```python
from build123d import *

# Parameters (mm, degrees)
SKETCH2_W                    = 37
SKETCH2_H                    = 30
BASE_FLANGE1_DEPTH           = 0.635
EDGE_FLANGE1_STRIP_W         = 4.0132
EDGE_FLANGE1_STRIP_H         = 0.635
EDGE_FLANGE1_STRIP_CUT_DEPTH = 37
EDGE_FLANGE1_DEPTH           = 37
EDGE_FLANGE2_START           = -6.6891
EDGE_FLANGE2_DEPTH           = 5.3175
EDGE_FLANGE2_2_DEPTH         = 0.3175
EDGE_FLANGE2_START_2         = -6.3716
EDGE_FLANGE2_3_DEPTH         = 5
EDGE_FLANGE3_START           = -6.6891
EDGE_FLANGE3_DEPTH           = 5.3175
EDGE_FLANGE3_2_DEPTH         = 0.3175
EDGE_FLANGE3_START_2         = -6.3716
EDGE_FLANGE3_3_DEPTH         = 5
SKETCH14_R                   = 1.7
CUT_EXTRUDE1_DEPTH           = 10
FILLET1_R                    = 3
SKETCH15_R                   = 1.7
CUT_EXTRUDE2_DEPTH           = 10


# Read off the part's stored shape, not the designer's step: Edge-Flange2, Edge-Flange3
# Sheet-metal steps are written as plain solids
with BuildPart() as part:
    # Sketch2 → Base-Flange1 (new body)
    with BuildSketch(Plane(origin=(0, 0, 0), x_dir=(0, 0, -1), z_dir=(1, 0, 0))):
        with Locations((18.5, -15)):
            Rectangle(SKETCH2_W, SKETCH2_H)
    extrude(amount=-BASE_FLANGE1_DEPTH)

    # Edge-Flange1 strip (across the edge) → Edge-Flange1 strip cut (cut)
    with BuildSketch(Plane(origin=(-0.635, 0, 0), x_dir=(0, -1, 0), z_dir=(0, 0, -1))):
        with Locations((-1.27, -0.3175)):
            Rectangle(EDGE_FLANGE1_STRIP_W, EDGE_FLANGE1_STRIP_H)
    extrude(amount=EDGE_FLANGE1_STRIP_CUT_DEPTH, mode=Mode.SUBTRACT)

    # Edge-Flange1 section (across the edge) → Edge-Flange1 (add)
    with BuildSketch(Plane(origin=(-0.635, 0, 0), x_dir=(0, -1, 0), z_dir=(0, 0, -1))):
        with BuildLine():
            Line((-0.635, 0.7366), (-0.635, 22))
            Line((-0.635, 22), (0, 22))
            Line((0, 22), (0, 0.7366))
            ThreePointArc((0, 0.7366), (0.215745145, 0.215745145), (0.7366, 0))
            Line((0.7366, 0), (0.7366, -0.635))
            ThreePointArc((0.7366, -0.635), (-0.233267661, -0.233267661), (-0.635, 0.7366))
        make_face()
    extrude(amount=EDGE_FLANGE1_DEPTH)

    # Edge-Flange2 outline → Edge-Flange2 (cut)
    with BuildSketch(Plane.YZ.offset(EDGE_FLANGE2_START)):
        with BuildLine():
            Line((0, 0), (0, -0.214574936))
            ThreePointArc((0, -0.214574936), (0.465815718, -0.711688642), (0.635, -1.3716))
            Line((0.635, -1.3716), (0.635, 0))
            Line((0.635, 0), (0, 0))
        make_face()
    extrude(amount=EDGE_FLANGE2_DEPTH, mode=Mode.SUBTRACT)

    # Edge-Flange2 2 outline → Edge-Flange2 2 (cut)
    with BuildSketch(Plane.YZ.offset(EDGE_FLANGE2_START)):
        with BuildLine():
            ThreePointArc((0.635, -1.3716), (0.465815718, -0.711688642), (0, -0.214574936))
            Line((0, -0.214574936), (0, -1.6891))
            Line((0, -1.6891), (0.635, -1.6891))
            Line((0.635, -1.6891), (0.635, -1.3716))
        make_face()
    extrude(amount=EDGE_FLANGE2_2_DEPTH, mode=Mode.SUBTRACT)

    # Edge-Flange2 3 outline → Edge-Flange2 3 (add)
    with BuildSketch(Plane.YZ.offset(EDGE_FLANGE2_START_2)):
        with BuildLine():
            Line((-0.7366, 0), (-8, 0))
            Line((-8, 0), (-8, -0.635))
            Line((-8, -0.635), (-0.7366, -0.635))
            ThreePointArc((-0.7366, -0.635), (-0.215745145, -0.850745145), (0, -1.3716))
            Line((0, -1.3716), (0, -0.214574936))
            ThreePointArc((0, -0.214574936), (-0.352991488, -0.054735896), (-0.7366, 0))
        make_face()
    extrude(amount=EDGE_FLANGE2_3_DEPTH)

    # Edge-Flange3 outline → Edge-Flange3 (cut)
    with BuildSketch(Plane.YZ.offset(EDGE_FLANGE3_START)):
        with BuildLine():
            ThreePointArc((0.635, -35.6284), (0.465815718, -36.288311358), (0, -36.785425064))
            Line((0, -36.785425064), (0, -37))
            Line((0, -37), (0.635, -37))
            Line((0.635, -37), (0.635, -35.6284))
        make_face()
    extrude(amount=EDGE_FLANGE3_DEPTH, mode=Mode.SUBTRACT)

    # Edge-Flange3 2 outline → Edge-Flange3 2 (cut)
    with BuildSketch(Plane.YZ.offset(EDGE_FLANGE3_START)):
        with BuildLine():
            Line((0, -35.3109), (0, -36.785425064))
            ThreePointArc((0, -36.785425064), (0.465815718, -36.288311358), (0.635, -35.6284))
            Line((0.635, -35.6284), (0.635, -35.3109))
            Line((0.635, -35.3109), (0, -35.3109))
        make_face()
    extrude(amount=EDGE_FLANGE3_2_DEPTH, mode=Mode.SUBTRACT)

    # Edge-Flange3 3 outline → Edge-Flange3 3 (add)
    with BuildSketch(Plane.YZ.offset(EDGE_FLANGE3_START_2)):
        with BuildLine():
            Line((-8, -37), (-0.7366, -37))
            ThreePointArc((-0.7366, -37), (-0.352991488, -36.945264104), (0, -36.785425064))
            Line((0, -36.785425064), (0, -35.6284))
            ThreePointArc((0, -35.6284), (-0.215745145, -36.149254855), (-0.7366, -36.365))
            Line((-0.7366, -36.365), (-8, -36.365))
            Line((-8, -36.365), (-8, -37))
        make_face()
    extrude(amount=EDGE_FLANGE3_3_DEPTH)

    # Sketch14 → Cut-Extrude1 (cut)
    with BuildSketch(Plane(origin=(0, 0, 0), x_dir=(0, 0, -1), z_dir=(1, 0, 0))):
        with Locations((3.5, -20)):
            Circle(SKETCH14_R)
        with Locations((33.5, -20)):
            Circle(SKETCH14_R)
    extrude(amount=-CUT_EXTRUDE1_DEPTH, mode=Mode.SUBTRACT)

    # Fillet1
    fillet1_edges = [part.edges().sort_by_distance(p)[0] for p in [
        (-22.635, 0.3175, 0),
        (-22.635, 0.3175, -37),
        (-0.3175, -30, -37),
        (-0.3175, -30, 0),
    ]]
    fillet(fillet1_edges, radius=FILLET1_R)

    # Sketch15 → Cut-Extrude2 (cut)
    with BuildSketch(Plane(origin=(0, 0.635, 0), x_dir=(1, 0, 0), z_dir=(0, 1, 0))):
        with Locations(Location((-12.635, 30.5, 0), (0, 0, 180))):
            Circle(SKETCH15_R)
        with Locations(Location((-12.635, 6.5, 0), (0, 0, 180))):
            Circle(SKETCH15_R)
    extrude(amount=-CUT_EXTRUDE2_DEPTH, mode=Mode.SUBTRACT)


solid = part.part
```
Geometry: final body of the model. Coordinates: model frame, mm. A direction names the side the tool comes from. Coordinates: 2 decimals unless noted, no trailing zeros. Order: outer loops, then holes, each group sorted by start corner. A loop starts at its lowest first (then second) coordinate and runs counter-clockwise, first axis right, second up. Notation, with made-up numbers: (65, -13) -> (105, -13) arc R22 cw to (105, 17) -> close; hole circle Ø6 at (-28.75, -10.5). An arc over 180 degrees is marked (long way). Write each question's results on one line, items separated by ' | '. Start each with the question number.
1) Cut plane B-B, the plane z = -33.5. Output: boundary loops of the cut face in (x, y) (3 decimals).
2) Cut plane C-C, the plane x = -2.25. Output: boundary loops of the cut face in (y, z) (3 decimals).
3) First-contact query: pin 1 (10 mm diameter, centred on x = -18.5, z = -18.5, fed in from -Y); pin 2 (1.4 mm diameter, centred on y = -4, z = -36, fed in from -X); pin 3 (12 mm diameter, centred on y = -9.5, z = -26.5, fed in from -X) (3 decimals); pin 4 (3 mm diameter, centred on y = -20, z = -33.5, fed in from +X). Flat tips, straight axial feed; report the tip coordinate or a pass-through.
4) Set-up query: faces 1 (the flat face through (-1.372, -4.1, -36.6)), 2 (the flat face through (-6.372, -2.78, -0.46)), 3 (the flat face through (-4, -4, -36.365)), 4 (the flat face through (-4, -4, -37)). Return all of +Z, -Z, +X, -X, +Y, -Y with unobstructed straight access to the full face (end or side cutting, diameter ignored); none if empty.
5) Mould query, pull axis X, two halves, no side actions, for faces 5 (the cylindrical face through (-13.42, 0.32, -32.01)), 6 (the cylindrical face through (-21.733, 0.313, -36.145)), 7 (the flat face through (-0.4, -13.4, 0)). Classes: released by +X, released by -X, zero draft, split by the parting line, or undercut.
6) Cut plane A-A, the plane y = -20. Output: boundary loops of the cut face in (x, z) (3 decimals).
7) Cut plane D-D, the plane y = -5.5. Output: boundary loops of the cut face in (x, z) (3 decimals), and give its area (3 significant figures).
8) Material intervals for line 1 along Y through (x, z) = (-0.2, -3.5); line 2 along X through (y, z) = (-22, -32) (3 decimals); line 3 along Y through (x, z) = (-0.35, -33.5), sorted ascending.
Checks:
1) outline: (-22.635, 0) -> (-1.372, 0) arc R0.737 cw to (-0.635, -0.737) -> (-0.635, -18.3) -> (0, -18.3) -> (0, -0.737) arc R1.372 ccw to (-1.372, 0.635) -> (-22.635, 0.635) -> close; (-0.635, -30) -> (0, -30) -> (0, -21.7) -> (-0.635, -21.7) -> close
2) outline: (-8, -37) -> (-0.737, -37) arc R1.372 ccw to (0.635, -35.628) -> (0.635, -1.372) arc R1.372 ccw to (-0.737, 0) -> (-8, 0) -> (-8, -0.635) -> (-0.737, -0.635) arc R0.737 cw to (0, -1.372) -> (0, -35.628) arc R0.737 cw to (-0.737, -36.365) -> (-8, -36.365) -> close
3) pin 1: y = 0 | pin 2: x = -6.37 | pin 3: x = -0.635 | pin 4: through
4) face 1: +Z, -Z, -Y | face 2: +Z, +Y, -Y | face 3: -X, -Y | face 4: -Z, +X, -X, +Y, -Y
5) face 5: undercut | face 6: released by -X | face 7: zero draft
6) outline: (-0.635, -37) -> (0, -37) -> (0, -35.2) -> (-0.635, -35.2) -> close; (-0.635, -31.8) -> (0, -31.8) -> (0, -5.2) -> (-0.635, -5.2) -> close; (-0.635, -1.8) -> (0, -1.8) -> (0, 0) -> (-0.635, 0) -> close
7) outline: (-6.372, -37) -> (-1.372, -37) -> (-1.372, -36.365) -> (-6.372, -36.365) -> close; (-6.372, -0.635) -> (-1.372, -0.635) -> (-1.372, 0) -> (-6.372, 0) -> close; (-0.635, -37) -> (0, -37) -> (0, 0) -> (-0.635, 0) -> close | area: 29.8 mm^2
8) line 1: -30 to -21.7, -18.3 to -0.02 | line 2: -0.635 to 0 | line 3: -30 to -21.7, -18.3 to 0.18
